```python
from build123d import *

# Parameters (mm, degrees)
F0_R     = 1.75
F0_R_2   = 11
F1_DEPTH = 40


with BuildPart() as f1:
    # F0 (on Right) → F1 (new body)
    with BuildSketch(Plane.YZ):
        Polygon((-46.3, -37.3), (-41.3, -42.3), (-9.15, -42.3), (-4, -37.3), (-4, -5), (-9.15, 0), (-41.3, 0), (-46.3, -5), align=None)
        with Locations((-40.725, -36.65)):
            Circle(F0_R, mode=Mode.SUBTRACT)
        with Locations((-9.725, -36.65)):
            Circle(F0_R, mode=Mode.SUBTRACT)
        with Locations((-40.725, -5.65)):
            Circle(F0_R, mode=Mode.SUBTRACT)
        with Locations((-25.15, -21.15)):
            Circle(F0_R_2, mode=Mode.SUBTRACT)
        with Locations((-9.725, -5.65)):
            Circle(F0_R, mode=Mode.SUBTRACT)
    extrude(amount=-F1_DEPTH)


solid = f1.part
```
Verification items for the finished model (mm, model axes). Coordinates: 2 decimals unless noted, no trailing zeros. Loops run counter-clockwise (first coordinate to the right, second up) from the corner with the lowest first, then second, coordinate; pieces in that order, holes last. Notation, with made-up numbers: (20, -16) - (70, -16) arc R28 ccw to (70, 16) - close; hole circle Ø3 at (-12.5, -35). An arc over 180 degrees is marked (long way). Answer as a JSON object with one key per item and string values.
(1) Go/stop test with flat-tipped pins: pin 1 Ø3 at (y, z) = (-40.725, -5.65) entering from -X; pin 2 Ø4 at (y, z) = (-40.725, -36.65) entering from +X. Record where each tip stops, or that it passes through.
Response:
{"pin 1": "passes through", "pin 2": "stops at x = 0"}
(2) Cross-section at C-C, the plane y = -25.15. Record the boundary of the cut face in (x, z).
Response:
{"outline": "(-40, -42.3) - (0, -42.3) - (0, -32.15) - (-40, -32.15) - close; (-40, -10.15) - (0, -10.15) - (0, 0) - (-40, 0) - close"}
(3) Cross-section at D-D, the plane x = -13.5. Record the boundary of the cut face in (y, z) (3 decimals).
Response:
{"outline": "(-46.3, -37.3) - (-41.3, -42.3) - (-9.15, -42.3) - (-4, -37.3) - (-4, -5) - (-9.15, 0) - (-41.3, 0) - (-46.3, -5) - close; hole circle Ø3.5 at (-40.725, -36.65); hole circle Ø3.5 at (-40.725, -5.65); hole circle Ø22 at (-25.15, -21.15); hole circle Ø3.5 at (-9.725, -36.65); hole circle Ø3.5 at (-9.725, -5.65)"}
(4) Cross-section at B-B, the plane z = -36.65. Record the boundary of the cut face in (x, y) (3 decimals), then the cut area to 3 significant figures.
Response:
{"outline": "(-40, -46.3) - (0, -46.3) - (0, -42.475) - (-40, -42.475) - close; (-40, -38.975) - (0, -38.975) - (0, -11.475) - (-40, -11.475) - close; (-40, -7.975) - (0, -7.975) - (0, -4) - (-40, -4) - close", "area": "1,410 mm²"}
(5) Mould release check, pull along Y, two halves, no side actions. Record for faces 1 (the cylindrical face through (-19.72, -42.473, -5.573)), 2 (the cylindrical face through (-19.72, -42.114, -37.715)), 3 (the flat face through (-19.72, -6.539, -2.535)), 4 (the flat face through (-20, -25, 0)): pulls with the +Y half, pulls with the -Y half, needs draft (parallel to the pull), parting line crosses it, or undercut.
Response:
{"face 1": "undercut", "face 2": "undercut", "face 3": "pulls with the +Y half", "face 4": "needs draft"}
(6) Scan lines: line 1 along Z through (x, y) = (-11.5, -40); line 2 along Y through (x, z) = (-3, -37); line 3 along Y through (x, z) = (-16, -21). Record each from-to range of solid material in increasing order.
Response:
{"line 1": "z = -42.3 to -38.24, -35.06 to -7.24, -4.06 to 0", "line 2": "y = -46.3 to -42.44, -39.01 to -11.44, -8.01 to -4", "line 3": "y = -46.3 to -36.15, -14.15 to -4"}
(7) Cross-section at A-A, the plane z = -21.15. Record the boundary of the cut face in (x, y), then the cut area to 3 significant figures.
Response:
{"outline": "(-40, -46.3) - (0, -46.3) - (0, -36.15) - (-40, -36.15) - close; (-40, -14.15) - (0, -14.15) - (0, -4) - (-40, -4) - close", "area": "812 mm²"}
